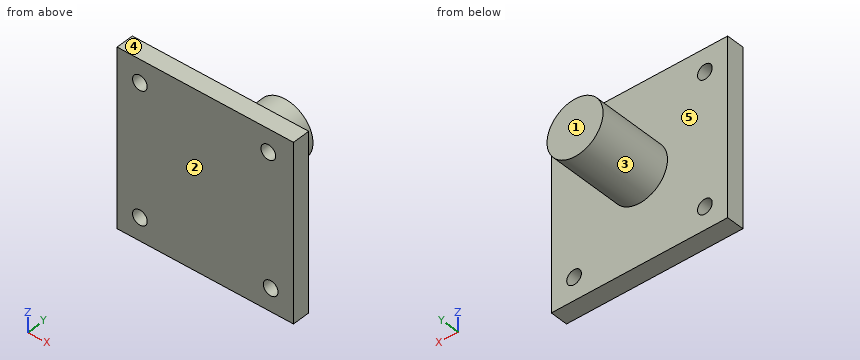
Autodesk Inventor part; units mm, degrees
ref_plane "YZ Plane" through (0, 0, 0) normal (1, 0, 0) x (0, 1, 0)
ref_plane "XZ Plane" through (0, 0, 0) normal (0, 1, 0) x (-1, 0, 0)
ref_plane "XY Plane" through (0, 0, 0) normal (0, 0, 1) x (1, 0, 0)
sketch "Boceto1" plane through (0, 0, 0) normal (0, 1, 0) x (-1, 0, 0)
  circle A0 centre (0, 0) radius 19.05
  line L0 (0, 0) -> (0, 22.5) construction
  line L1 (0, 22.5) -> (-32.5, 22.5) construction
  line L2 (-32.5, 22.5) -> (32.5, 22.5)
  line L3 (32.5, 22.5) -> (32.5, -22.5)
  line L4 (32.5, -22.5) -> (-32.5, -22.5)
  line L5 (-32.5, -22.5) -> (-32.5, 22.5)
  dimension "d0" = 38.1
  dimension "d1" = 22.5
  dimension "d2" = 32.5
  dimension "d3" = 65
  dimension "d4" = 45
extrude "Extrusión1" add sketch "Boceto1" along normal blind 50.8 contours A0
sketch "Boceto2" plane through (0, 0, 0) normal (0, -1, 0) x (1, 0, 0)
  line L0 (0, 0) -> (-60, 0) construction
  line L1 (-60, 0) -> (-60, -60) construction
  line L2 (-60, -60) -> (60, -60)
  line L3 (60, -60) -> (60, 60)
  line L4 (60, 60) -> (-60, 60)
  line L5 (-60, 60) -> (-60, -60)
  dimension "d7" = 60
  dimension "d8" = 60
  dimension "d9" = 120
  dimension "d10" = 120
extrude "Extrusión2" add sketch "Boceto2" along normal blind 12
thread "Rosca1"
sketch "Sketch4" plane through (0, 0, 0) normal (0, 1, 0) x (1, 0, 0)
  line L0 (60, 60) -> (60, -60) construction
  line L1 (-60, 60) -> (60, 60) construction
  line L2 (-60, -60) -> (-60, 60) construction
  line L3 (60, -60) -> (-60, -60) construction
  circle A0 centre (0, 0) radius 19.05 construction
  line L4 (-60, 60) -> (60, 60) construction
  line L5 (0, 60) -> (0, -60) construction
  line L6 (60, 60) -> (60, -60) construction
  line L7 (60, 0) -> (-60, 0) construction
  point P0 (-44.5, 44.5)
  point P1 (44.5, 44.5)
  point P2 (-44.5, -44.5)
  point P3 (42.8657, -44.5)
  dimension "d34" = 89
  dimension "d35" = 89
  dimension "d36" = 89
hole "Hole1" at (-44.5, 0, -44.5) at (44.5, 0, -44.5) at (-44.5, 0, 44.5) at (42.8657, 0, 44.5) direction (0, -1, 0) diameter 10 end through all
equation "\"d7\" = 0.5 * d9"
equation "\"d8\" = 0.5 * d10"
properties part number "conector cardan"
Geometry check sheet. Reference: the model listing, model coordinates, mm. Face numbers are marked on the shaded views. A direction names the side the tool comes from. Coordinates: 2 decimals unless noted, no trailing zeros. Order: outer loops, then holes, each group sorted by start corner. A loop starts at its lowest first (then second) coordinate and runs counter-clockwise, first axis right, second up.
Q1. Tool access check on the marked faces 4 and 5. Record the directions out of +Z, -Z, +X, -X, +Y, -Y that give a thin tool (end or side, any length) a straight path to the whole face; none if there is none.
Reply:
face 4: +Z, +X, -X, +Y, -Y
face 5: +Y
Q2. Sectioned sample at C-C on x = 0. Record the cut outline in (y, z).
Reply:
outline: (-12, -60) - (0, -60) - (0, -19.05) - (50.8, -19.05) - (50.8, 19.05) - (0, 19.05) - (0, 60) - (-12, 60) - close
Q3. Sectioned sample at A-A on x = -44.5. Record the cut outline in (y, z).
Reply:
outline: (-12, -60) - (0, -60) - (0, -49.5) - (-12, -49.5) - close; (-12, -39.5) - (0, -39.5) - (0, 39.5) - (-12, 39.5) - close; (-12, 49.5) - (0, 49.5) - (0, 60) - (-12, 60) - close
Q4. Draft check along Y on the marked faces 1, 2 and 3. Enter one of: released by +Y, released by -Y, zero draft, split by the parting line, or undercut.
Reply:
face 1: released by +Y
face 2: released by -Y
face 3: zero draft
Q5. Thickness scan on probe 1 along X at (y, z) = (-7, 44.5); probe 2 along X at (y, z) = (-8, 44); probe 3 along Z at (x, y) = (-44.5, -5.75). Record the ranges inside material, lowest first.
Reply:
probe 1: x = -60 to -49.5, -39.5 to 37.87, 47.87 to 60
probe 2: x = -60 to -49.47, -39.53 to 37.89, 47.84 to 60
probe 3: z = -60 to -49.5, -39.5 to 39.5, 49.5 to 60
Q6. Sectioned sample at B-B on z = -44.5. Record the cut outline in (x, y), and give its area (3 significant figures).
Reply:
outline: (-60, -12) - (-49.5, -12) - (-49.5, 0) - (-60, 0) - close; (-39.5, -12) - (39.5, -12) - (39.5, 0) - (-39.5, 0) - close; (49.5, -12) - (60, -12) - (60, 0) - (49.5, 0) - close
area: 1,200 mm2
Q7. Sectioned sample at D-D on y = 15. Record the cut outline in (x, z), and give its area (3 significant figures).
Reply:
outline: circle Ø38.1 at (0, 0)
area: 1,140 mm2
Q8. Depth check by flat-ended pin: pin 1 Ø9 at (x, z) = (-44.5, -44.5) entering from -Y; pin 2 Ø6 at (y, z) = (29.5, 20) entering from -X; pin 3 Ø11.5 at (x, z) = (44.5, -44.5) entering from +Y; pin 4 Ø12 at (y, z) = (38, -2.5) entering from -X. Enter the tip coordinate at first touch or a pass-through.
Reply:
pin 1: passes through
pin 2: stops at x = -8.6
pin 3: stops at y = 0
pin 4: stops at x = -19.05
